Build history of the part. All positions in model axes, mm. Face numbers are marked on the shaded views. A direction names the side the tool comes from. Coordinates: 2 decimals unless noted, no trailing zeros. Loops run counter-clockwise (first coordinate to the right, second up) from the corner with the lowest first, then second, coordinate; pieces in that order, holes last.
(1) Slice it at C-C (y = 7.5). Give the cut face in (x, z), and give its area (3 significant figures).
(2) Tool access for the marked faces 4 and 5: list every direction of +Z, -Z, +X, -X, +Y, -Y with a clear straight run to the whole face (end or side of a thin tool).
(3) Slice it at B-B (x = 15.5). Give the cut face in (y, z), and give its area (3 significant figures).
(4) Slice it at D-D (z = 8). Give the cut face in (x, y), and give its area (3 significant figures).
(5) Flat gauge pins, fed straight in: P1, Ø3.5, axis at x = -6, y = 18, coming from the -Z side; P2, Ø2.5, axis at y = 4, z = 79.5, coming from the -X side; P3, Ø13, axis at x = -10, y = 21, coming from the +Z side. Where does each tip first touch, or does it go through?
(6) Two-plate mould, pull along X, no slides. Class the marked faces 1, 2 and 3: pulls with the +X half, pulls with the -X half, needs draft (parallel to the pull), parting line crosses it, or undercut.
(7) Wall check: L1, parallel to Z at x = 61, y = 16; L2, parallel to X at y = 30, z = 31; L3, parallel to Y at x = -1.1, z = 29.7. Give the ranges that are in metal, low to high.
Autodesk Inventor part; units mm, degrees
ref_plane "YZ Plane" through (0, 0, 0) normal (1, 0, 0) x (0, 1, 0)
ref_plane "XZ Plane" through (0, 0, 0) normal (0, 1, 0) x (-1, 0, 0)
ref_plane "XY Plane" through (0, 0, 0) normal (0, 0, 1) x (1, 0, 0)
sketch "Sketch1" plane through (0, 0, 0) normal (0, 1, 0) x (-1, 0, 0)
  line L0 (0, 0) -> (-111, 0)
  line L1 (-111, 0) -> (-111, 82)
  line L2 (-111, 82) -> (0, 82)
  line L3 (0, 82) -> (0, 0)
  dimension "d0" = 111
  dimension "d1" = 82
extrude "Extrusion1" add sketch "Sketch1" along normal blind 2
sketch "Sketch2" plane through (0, 0, 0) normal (0, -1, 0) x (1, 0, 0)
  point P0 (0, 0)
sketch "Sketch3" plane through (0, 0, 0) normal (0, -1, 0) x (1, 0, 0)
  line L0 (0, 0) -> (0, 82)
  line L1 (0, 0) -> (0, 82)
  line L2 (0, 82) -> (-2, 82)
  line L3 (-2, 82) -> (-2, 0)
  line L4 (-2, 0) -> (0, 0)
  line L5 (-2, 0) -> (-2, -2)
  line L6 (-2, -2) -> (113, -2)
  line L7 (113, -2) -> (113, 0)
  line L8 (113, 0) -> (-2, 0)
  line L9 (113, 0) -> (113, 84)
  line L10 (113, 84) -> (111, 84)
  line L11 (111, 84) -> (111, -2)
  line L12 (111, 84) -> (-2, 84)
  line L13 (111, 82) -> (111, 0)
  line L14 (-2, 82) -> (111, 82)
  line L15 (111, 82) -> (111, 84)
  dimension "d4" = 2
  dimension "d5" = 2
  dimension "d6" = 115
  dimension "d7" = 2
  dimension "d8" = 84
  dimension "d9" = 2
extrude "Extrusion2" add sketch "Sketch3" against normal blind 50 contours L11 L10 L9 L8
sketch "Sketch4" plane through (0, 0, 0) normal (0, -1, 0) x (1, 0, 0)
  line L0 (111, 84) -> (111, 82)
  line L1 (111, 84) -> (-2, 84)
  line L2 (-2, 84) -> (-2, 82)
  line L3 (0, 82) -> (111, 82)
  line L4 (-2, 82) -> (111, 82)
  line L5 (111, 82) -> (111, 84)
  point P0 (0, 0)
  dimension "d12" = 113
extrude "Extrusion3" add sketch "Sketch4" against normal blind 50
sketch "Sketch5" plane through (0, 0, 0) normal (0, -1, 0) x (1, 0, 0)
  line L0 (-2, 84) -> (-2, 82)
  line L1 (-2, 82) -> (-2, -2)
  line L2 (-2, -2) -> (0, -2)
  line L3 (0, 0) -> (0, 82)
  line L4 (0, -2) -> (0, 82)
  line L5 (-2, 82) -> (0, 82)
  line L6 (0, 82) -> (-2, 82)
  dimension "d15" = 84
extrude "Extrusion4" add sketch "Sketch5" against normal blind 50
sketch "Sketch6" plane through (0, 0, 0) normal (0, -1, 0) x (1, 0, 0)
  line L0 (0, 0) -> (113, 0)
  line L1 (113, 0) -> (113, -2)
  line L2 (0, 82) -> (0, -2)
  line L3 (113, -2) -> (0, -2)
  line L4 (0, -2) -> (0, 0)
  dimension "d18" = 2
extrude "Extrusion5" add sketch "Sketch6" against normal blind 50
sketch "Sketch7" plane through (-2, 0, 84) normal (-1, 0, 0) x (0, 0, 1)
  circle A0 centre (-54.3, 17.5) radius 2.5
  point P0 (-84, 0)
  dimension "d21" = 5
hole "Hole1" at (-2, 17.5, 29.7) direction (1, 0, 0) diameter 5 depth 2 tip angle 118
sketch "Sketch8" plane through (-2, 0, 84) normal (-1, 0, 0) x (0, 0, 1)
  line L0 (-61.8, 10) -> (-61.8, 25)
  line L1 (-61.8, 25) -> (-46.8, 25)
  line L2 (-46.8, 25) -> (-46.8, 10)
  line L3 (-46.8, 10) -> (-61.8, 10)
  point P0 (-84, 0)
  dimension "d29" = 15
  dimension "d30" = 15
  dimension "d31" = 15
extrude "Extrusion6" add sketch "Sketch8" along normal blind 12
chamfer "Chamfer1" distance 10 angle 45 1 edges at (-14, 25, 29.7)
sketch "Sketch9" plane through (-2, 10, 22.2) normal (0, -1, 0) x (1, 0, 0)
  line L0 (0, 0) -> (0, 15)
  line L1 (0, 2) -> (-10, 2)
  line L2 (-12, 0) -> (-12, 15)
  line L3 (-10, 2) -> (-10, 13)
  line L4 (0, 15) -> (-12, 15)
  line L5 (-10, 13) -> (0, 13)
  line L6 (0, 13) -> (0, 2)
  point P0 (2, -22.2)
  point P1 (0, 13)
  dimension "d37" = 10
  dimension "d38" = 11
extrude "Extrusion7" cut sketch "Sketch9" against normal blind 13
sketch "Sketch10" plane through (-14, 15, 22.2) normal (-0.7071, 0.7071, 0) x (-0.7071, -0.7071, 0)
  line L0 (-14.1421, 15) -> (-14.1421, 0)
  line L1 (-14.1421, 0) -> (-14.1421, 15)
  line L2 (0, 0) -> (0, 15)
  line L3 (-14.1421, 15) -> (0, 15)
  line L4 (0, 15) -> (0, 0)
  line L5 (-14.1421, 0) -> (0, 0)
  line L6 (0, 0) -> (-14.1421, 0)
  point P0 (0.7071, -22.2)
extrude "Extrusion8" add sketch "Sketch10" along normal blind 2
chamfer "Chamfer2" distance 2 angle 45 1 edges at (-5.4142, 26.4142, 29.7)
chamfer "Chamfer3" distance 2 angle 45 1 edges at (-15.4142, 16.4142, 29.7)
sketch "Sketch11" plane through (0, 2, 0) normal (0, 1, 0) x (1, 0, 0)
  line L0 (0, 0) -> (0, -82)
  line L1 (0, 0) -> (0, -6)
  line L2 (0, -6) -> (6, -6)
  line L3 (6, -6) -> (6, 0)
  line L4 (0, 0) -> (111, 0)
  line L5 (6, 0) -> (0, 0)
  dimension "d49" = 6
  dimension "d50" = 6
  dimension "d51" = 6
extrude "Extrusion9" add sketch "Sketch11" along normal blind 3
sketch "Sketch12" plane through (0, 2, 0) normal (0, 1, 0) x (1, 0, 0)
  point P0 (0, 0)
sketch "Sketch13" plane through (0, 2, 0) normal (0, 1, 0) x (1, 0, 0)
  line L0 (111, 0) -> (111, -6)
  line L1 (111, 0) -> (111, -82)
  line L2 (111, -6) -> (105, -6)
  line L3 (105, -6) -> (105, 0)
  line L4 (0, 0) -> (111, 0)
  line L5 (105, 0) -> (111, 0)
  dimension "d54" = 6
  dimension "d55" = 6
extrude "Extrusion10" add sketch "Sketch13" along normal blind 3
sketch "Sketch14" plane through (0, 2, 0) normal (0, 1, 0) x (1, 0, 0)
  point P0 (0, 0)
sketch "Sketch15" plane through (0, 2, 0) normal (0, 1, 0) x (1, 0, 0)
  line L0 (0, -82) -> (111, -82)
  line L1 (0, -82) -> (0, -76)
  line L2 (0, -6) -> (0, -82)
  line L3 (0, -76) -> (6, -76)
  line L4 (6, -76) -> (6, -82)
  point P0 (0, 0)
  dimension "d58" = 6
  dimension "d59" = 6
extrude "Extrusion11" add sketch "Sketch15" along normal blind 3
sketch "Sketch16" plane through (0, 2, 0) normal (0, 1, 0) x (1, 0, 0)
  line L0 (111, -82) -> (0, -82)
  line L1 (111, -82) -> (111, -76)
  line L2 (111, 0) -> (111, -82)
  line L3 (111, -76) -> (105, -76)
  line L4 (105, -76) -> (105, -82)
  line L5 (105, -82) -> (111, -82)
  point P0 (0, 0)
  dimension "d62" = 6
  dimension "d63" = 6
extrude "Extrusion12" add sketch "Sketch16" along normal blind 3
properties part number "box"
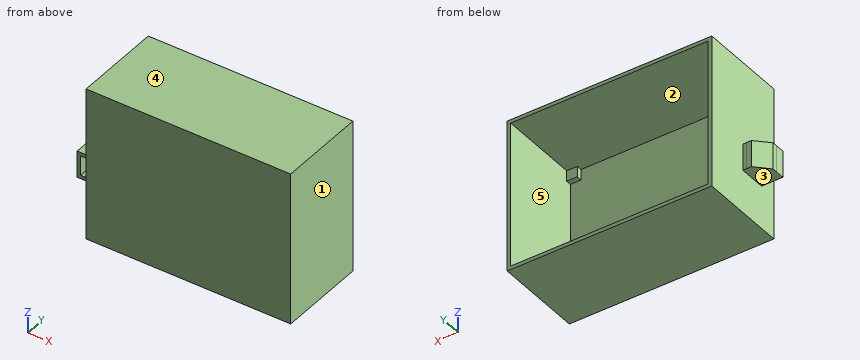
Response values:
1. outline: (-2, -2) - (113, -2) - (113, 84) - (-2, 84) - close; hole (0, 0) - (111, 0) - (111, 82) - (0, 82) - close
1. area: 788 mm2
2. face 4: +Z, +X, -X, +Y, -Y
2. face 5: +Y
3. outline: (0, -2) - (50, -2) - (50, 0) - (2, 0) - (2, 82) - (50, 82) - (50, 84) - (0, 84) - close
3. area: 364 mm2
4. outline: (-2, 0) - (113, 0) - (113, 50) - (111, 50) - (111, 2) - (0, 2) - (0, 50) - (-2, 50) - close
4. area: 422 mm2
5. P1: stops at z = 22.2
5. P2: stops at x = -2
5. P3: stops at z = 37.2
6. face 1: pulls with the +X half
6. face 2: undercut
6. face 3: needs draft
7. L1: z = -2 to 0, 82 to 84
7. L2: x = -2 to 0, 111 to 113
7. L3: y = 0 to 15, 20 to 50
